Solid Edge part; units mm, degrees
sketch "Sketch1" plane through (0, 0, 0) normal (0, -1, 0) x (1, 0, 0)
  line L0 (0, 30) -> (0, 0)
  line L1 (0.75, 0) -> (0, 0)
  line L2 (0.75, -2.5) -> (0.75, 0)
  line L3 (0, -2.5) -> (0.75, -2.5)
  line L4 (0, -3) -> (0, -2.5)
  line L5 (1.5, -3) -> (0, -3)
  line L6 (1.5, 0) -> (1.5, -3)
  line L7 (2.5, 0) -> (1.5, 0)
  line L8 (2.5, 0) -> (2.5, 30)
  line L9 (2.5, 30) -> (0, 30)
extrude "Protrusion1" add sketch "Sketch1" against normal blind 80
sketch "Sketch2" plane through (1.25, 80, 13.5) normal (0, 1, 0) x (0, 0, 1)
  line L0 (15.5, -1.25) -> (15.5, 0)
  line L1 (15.5, 0) -> (14.5, 0)
  line L2 (14.5, 0) -> (14.5, -1.25)
extrude "Vyříznutí_1" cut sketch "Sketch2" against normal blind 110.5 material side at (0.625, 80, 28.95)
extrude "Protrusion2" [suppressed]
extrude "Cutout1" [suppressed]
extrude "Cutout2" [suppressed]
extrude "Cutout3" [suppressed]
extrude "Cutout4" [suppressed]
sketch "Sketch3" plane through (1.25, 40, 30) normal (0, 0, 1) x (0, 1, 0)
  line L0 (-38, 1.25) -> (-37, 1.25)
  line L1 (-37, 1.25) -> (-37, 0)
  line L2 (-37, 0) -> (-38, 0)
  line L3 (-38, 0) -> (-38, 1.25)
extrude "Cutout5" cut sketch "Sketch3" against normal blind 30
sketch "Sketch4" plane through (2.5, 40, 15) normal (1, 0, 0) x (0, 1, 0)
  line L0 (-27.8483, -0.3216) -> (-27.8483, 11.6784)
  line L1 (-27.8483, 11.6784) -> (-35.8483, 11.6784)
  line L2 (-35.8483, 11.6784) -> (-35.8483, -0.3216)
  line L3 (-35.8483, -0.3216) -> (-27.8483, -0.3216)
  line L4 (-27.8483, -12.9122) -> (-27.8483, -8.9122)
  line L5 (-27.8483, -8.9122) -> (-35.8483, -8.9122)
  line L6 (-35.8483, -8.9122) -> (-35.8483, -12.9122)
  line L7 (-35.8483, -12.9122) -> (-27.8483, -12.9122)
extrude "Vyříznutí_8" cut sketch "Sketch4" against normal blind 2.5
Could you check a few things on this model? Use its own coordinates, in mm. A direction names the side the tool comes from. Coordinates: 2 decimals unless noted, no trailing zeros. Write each loop counter-clockwise with the first axis right and the second up, starting at its lowest first coordinate (ties: lowest second). Pieces come first, ordered by that corner, then holes. Notation, with made-up numbers: (24.5, 5.5) - (76.5, 5.5) arc R15 cw to (76.5, 24.5) - close; hole circle Ø4 at (-33, 45). An arc over 180 degrees is marked (long way). Write item = value, one per line.
1) Will this pin go through, and if not, where does the flat tip stop? pin 1 Ø1.5 at (y, z) = (51.5, -2) entering from +X.
Result set:
pin_1 = 1.5
2) We'd pull the mould along Y, two halves only. Please class faces 1 (the flat face through (1, 8, 6.088)), 2 (the flat face through (1, 0, 14)), 3 (the flat face through (0, 41, 14)): +Y half, -Y half, draft (parallel to the pull), parting line (faces both ways), or undercut.
Result set:
face_1 = undercut
face_2 = -Y half
face_3 = draft
3) Please list where these lines run through material, in increasing order: line 1 (Z direction, x = 0.4, y = 73); line 2 (Y direction, x = 0.1, z = 25); line 3 (Y direction, x = 2.15, z = 4.5). Write a range as [from, to].
Result set:
line_1 = [-3, -2.5], [0, 28], [29, 30]
line_2 = [0, 2], [3, 4.15], [12.15, 80]
line_3 = [0, 4.15], [12.15, 80]
4) For faces 4 (the flat face through (1.5, 39, -1)), 5 (the flat face through (0, 1, 14)), 6 (the flat face through (0.75, 39, -1)), 7 (the flat face through (1, 12.152, 4)), which set-ups out of +Z, -Z, +X, -X, +Y, -Y let a thin tool reach every point of the face, with its end or its side?
Result set:
face_4 = -Z, +X, +Y, -Y
face_5 = +Z, -Z, -X, +Y, -Y
face_6 = -X, +Y, -Y
face_7 = +X, -X
5) Suppose I cut it at B-B on y = 5.5. Please give me the cut outline in (x, z), plus the area to 3 significant figures.
Result set:
outline = (0, -3) - (1.5, -3) - (1.5, 0) - (2.5, 0) - (2.5, 2.09) - (0, 2.09) - (0, 0) - (0.75, 0) - (0.75, -2.5) - (0, -2.5) - close; (0, 6.09) - (2.5, 6.09) - (2.5, 14.68) - (0, 14.68) - close; (0, 26.68) - (2.5, 26.68) - (2.5, 30) - (0, 30) - (0, 29) - (1.25, 29) - (1.25, 28) - (0, 28) - close
area = 36.4 mm2
6) Suppose I cut it at C-C on y = 39.5. Please give me the cut outline in (x, z), plus the area to 3 significant figures.
Result set:
outline = (0, -3) - (1.5, -3) - (1.5, 0) - (2.5, 0) - (2.5, 30) - (0, 30) - (0, 29) - (1.25, 29) - (1.25, 28) - (0, 28) - (0, 0) - (0.75, 0) - (0.75, -2.5) - (0, -2.5) - close
area = 76.4 mm2
7) Suppose I cut it at A-A on z = 4. Please give me the cut outline in (x, y).
Result set:
outline = (0, 0) - (2.5, 0) - (2.5, 4.15) - (0, 4.15) - (0, 3) - (1.25, 3) - (1.25, 2) - (0, 2) - close; (0, 12.15) - (2.5, 12.15) - (2.5, 80) - (0, 80) - close
